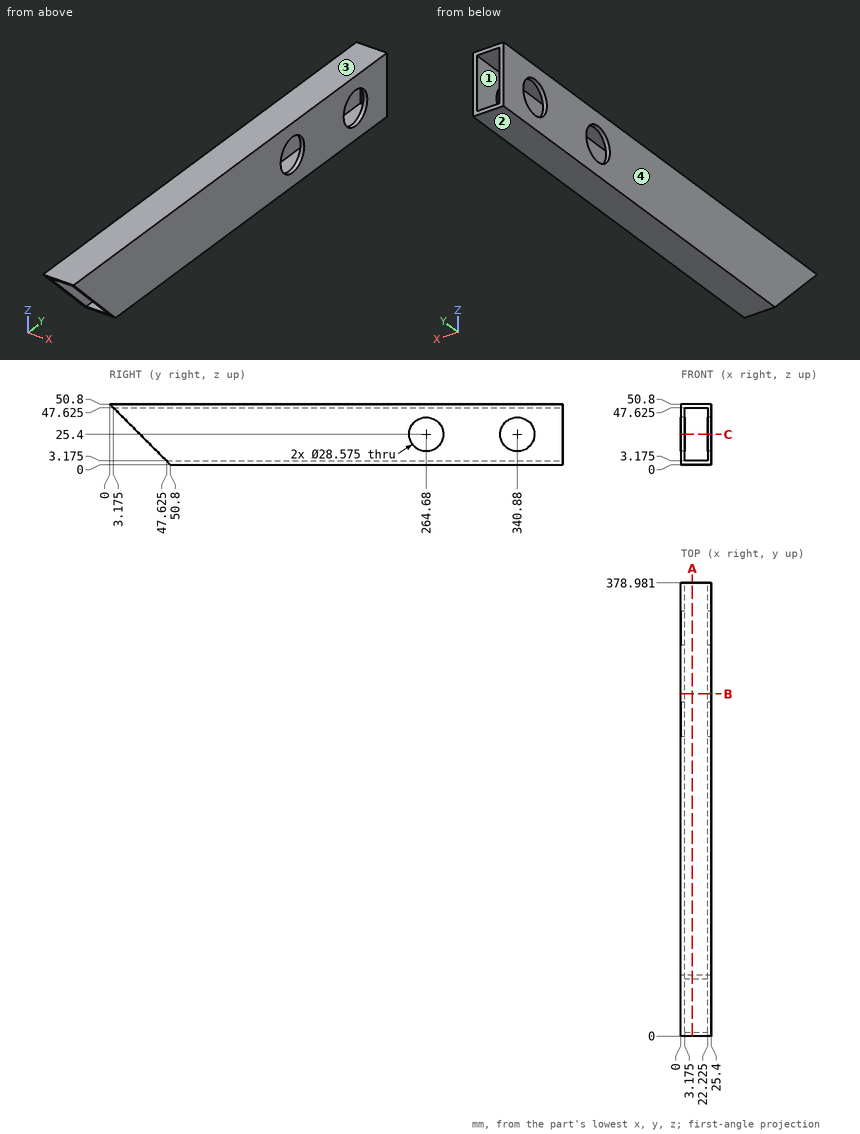
The drawing under review shows one solid part. Ordinate dimensions are in mm from its lowest x, y, z. Coordinates: 2 decimals unless noted, no trailing zeros. Loops run counter-clockwise (first coordinate to the right, second up) from the corner with the lowest first, then second, coordinate; pieces in that order, holes last. Notation, with made-up numbers: (-34.5, -19) - (5.5, -19) arc R26 ccw to (5.5, -3) - close; hole circle Ø9 at (24.5, 2). An arc over 180 degrees is marked (long way). Use CSV: the item, a comma, the result in double quotes. Start each with the question number.
1. Add section A-A on x = 9.5. Give the boundary of the cut face in (y, z) (1 decimal).
2. Mouldability with a two-part tool opening along Z and no side actions: class the marked faces 1, 2, 3 and 4 as released by +Z, released by -Z, zero draft, split by the parting line, or undercut.
3. To check wall thickness, follow probe 1 along Y at (x, z) = (1.7, 25.4) (1 decimal); probe 2 along X at (y, z) = (54, 9) (1 decimal); probe 3 along Z at (x, y) = (18.25, 88.5) (1 decimal). State the ranges of each line that lie inside material, in increasing order.
4. Add section C-C on z = 25.4. Give the boundary of the cut face in (x, y) (1 decimal), plus the area to 3 significant figures.
5. Clearance check with a flat-ended pin moving along its axis: pin 1 (12 mm diameter, centred on x = 12.5, z = 41, fed in from +Y). State where the tip first meets the part, or that it passes through.
6. Add section B-B on y = 286. Give the boundary of the cut face in (x, z) (1 decimal).
Resolved:
1,outline,"(0, 50.8) - (3.2, 47.6) - (379, 47.6) - (379, 50.8) - close; (47.6, 3.2) - (50.8, 0) - (379, 0) - (379, 3.2) - close"
2,face 1,"undercut"
2,face 2,"released by -Z"
2,face 3,"released by +Z"
2,face 4,"zero draft"
3,probe 1,"25.4 to 250.4, 279 to 326.6, 355.2 to 379"
3,probe 2,"0 to 3.2, 22.2 to 25.4"
3,probe 3,"0 to 3.2, 47.6 to 50.8"
4,outline,"(0, 25.4) - (3.2, 25.4) - (3.2, 250.4) - (0, 250.4) - close; (0, 279) - (3.2, 279) - (3.2, 326.6) - (0, 326.6) - close; (0, 355.2) - (3.2, 355.2) - (3.2, 379) - (0, 379) - close; (22.2, 25.4) - (25.4, 25.4) - (25.4, 250.4) - (22.2, 250.4) - close; (22.2, 279) - (25.4, 279) - (25.4, 326.6) - (22.2, 326.6) - close; (22.2, 355.2) - (25.4, 355.2) - (25.4, 379) - (22.2, 379) - close"
4,area,"1,880 mm2"
5,pin 1,"through"
6,outline,"(0, 0) - (25.4, 0) - (25.4, 50.8) - (0, 50.8) - close; hole (3.2, 3.2) - (22.2, 3.2) - (22.2, 47.6) - (3.2, 47.6) - close"
